```python
from build123d import *

# Parameters (mm, degrees)
SZKIC1_W                        = 2.5
SZKIC1_H                        = 20
WYTNIJ_WYCI_GNI_CIE1_DEPTH      = 10
WYTNIJ_WYCI_GNI_CIE1_DEPTH_BACK = 10
SZKIC3_R                        = 6.5
WYTNIJ_WYCI_GNI_CIE2_DEPTH      = 3.5
WYTNIJ_WYCI_GNI_CIE2_DEPTH_BACK = 3.5
SFAZOWANIE1_SIZE                = 1


with BuildPart() as part:
    # Szkic1 → Obrót1 (revolve)
    with BuildSketch(Plane(origin=(0, 0, 0), x_dir=(1, 0, 0), z_dir=(0, 1, 0))):
        with BuildLine():
            Line((0, 9), (0, -13))
            Line((0, -13), (2.5, -13))
            Line((2.5, -13), (7.636887524, -4.762137015))
            ThreePointArc((7.636887524, -4.762137015), (7.869537252, 4.366965014), (0, 9))
        make_face()
        with Locations((1.25, -23)):
            Rectangle(SZKIC1_W, SZKIC1_H)
    revolve(axis=Axis((0, 0, -26.043516498), (0, 0, 1)))

    # Szkic2 → Wytnij-wyciągnięcie1 (cut, two sides)
    with BuildSketch(Plane(origin=(0, 0, 0), x_dir=(0, 0, -1), z_dir=(1, 0, 0))) as wytnij_wyci_gni_cie1_sk:
        with BuildLine():
            Line((-13, 2.5), (8.645808233, 2.5))
            ThreePointArc((8.645808233, 2.5), (3.21988026, 8.4043067), (-4.762137015, 7.636887524))
            Line((-4.762137015, 7.636887524), (-13, 2.5))
        make_face()
        with BuildLine():
            Line((-13, -2.5), (8.645808233, -2.5))
            ThreePointArc((8.645808233, -2.5), (3.21988026, -8.4043067), (-4.762137015, -7.636887524))
            Line((-4.762137015, -7.636887524), (-13, -2.5))
        make_face()
    extrude(amount=WYTNIJ_WYCI_GNI_CIE1_DEPTH, mode=Mode.SUBTRACT)
    extrude(wytnij_wyci_gni_cie1_sk.sketch, amount=-WYTNIJ_WYCI_GNI_CIE1_DEPTH_BACK, mode=Mode.SUBTRACT)

    # Szkic3 → Wytnij-wyciągnięcie2 (cut, two sides)
    with BuildSketch(Plane(origin=(0, 0, 0), x_dir=(1, 0, 0), z_dir=(0, 1, 0))) as wytnij_wyci_gni_cie2_sk:
        Circle(SZKIC3_R)
    extrude(amount=WYTNIJ_WYCI_GNI_CIE2_DEPTH, mode=Mode.SUBTRACT)
    extrude(wytnij_wyci_gni_cie2_sk.sketch, amount=-WYTNIJ_WYCI_GNI_CIE2_DEPTH_BACK, mode=Mode.SUBTRACT)

    # Sfazowanie1
    sfazowanie1_edges = [part.edges().sort_by_distance(p)[0] for p in [
        (-2.5, 0, 33),
    ]]
    chamfer(sfazowanie1_edges, length=SFAZOWANIE1_SIZE)


solid = part.part
```
Geometry check sheet. Reference: the model listing, model coordinates, mm. A direction names the side the tool comes from. Coordinates: 2 decimals unless noted, no trailing zeros. Loops run counter-clockwise (first coordinate to the right, second up) from the corner with the lowest first, then second, coordinate; pieces in that order, holes last. Notation, with made-up numbers: (5, 36) -> (33, 36) arc R11 cw to (33, 46) -> close; hole circle Ø1 at (-23, -39.75). An arc over 180 degrees is marked (long way). Put each result on its own line as item: value.
1) Tool access check on faces 4 (the flat face through (0, 0, 33)), 5 (the cylindrical face through (-0.54, -2.44, 22.37)). Record the directions out of +Z, -Z, +X, -X, +Y, -Y that give a thin tool (end or side, any length) a straight path to the whole face; none if there is none.
Result set:
face 4: +Z, +X, -X, +Y, -Y
face 5: +Z
2) Release check for a two-part mould opening along X. For faces 1 (the cylindrical face through (-5.158, 0.035, 3.955)), 2 (the conical face through (4.53, -0.1, 9.74)), 3 (the flat face through (-3, -2.5, 6)) record: released by +X, released by -X, zero draft, split by the parting line, or undercut.
Result set:
face 1: undercut
face 2: released by +X
face 3: zero draft
3) Thickness scan on line 1 (X direction, y = -0.2, z = 0); line 2 (Z direction, x = 4, y = -1.9); line 3 (Z direction, x = -3.5, y = -0.5). Record the ranges inside material, lowest first.
Result set:
line 1: x = -9 to -6.5, 6.5 to 9
line 2: z = -7.84 to -5.12, 5.12 to 9.91
line 3: z = -8.28 to -5.48, 5.48 to 11.34
4) Cross-section at C-C on z = -5. Record the boundary of the cut face in (x, y).
Result set:
outline: (-7.05, -2.5) -> (-4.15, -2.5) -> (-4.15, 2.5) -> (-7.05, 2.5) arc R7.48 ccw to start; (4.15, -2.5) -> (7.05, -2.5) arc R7.48 ccw to (7.05, 2.5) -> (4.15, 2.5) -> close
5) Gauge pin test, flat end, axial feed: pin 1 Ø1.5 at (y, z) = (-1, 20) entering from +X. Record the tip position at first contact, or that the pin passes through.
Result set:
pin 1: stops at x = 2.49
6) Cross-section at B-B on y = 0. Record the boundary of the cut face in (x, z).
Result set:
outline: (-7.64, 4.76) arc R9 ccw (long way) to (7.64, 4.76) -> (2.5, 13) -> (2.5, 32) -> (1.5, 33) -> (-1.5, 33) -> (-2.5, 32) -> (-2.5, 13) -> close; hole circle Ø13 at (0, 0)
7) Cross-section at A-A on z = 0. Record the boundary of the cut face in (x, y).
Result set:
outline: (-8.65, -2.5) -> (-6.5, -2.5) -> (-6.5, 2.5) -> (-8.65, 2.5) arc R9 ccw to start; (6.5, -2.5) -> (8.65, -2.5) arc R9 ccw to (8.65, 2.5) -> (6.5, 2.5) -> close
